Here's how the part is built. I have some questions about the finished solid (model axes, mm). A direction names the side the tool comes from. Give positions to 0.01 mm unless a question says otherwise; leave off trailing zeros. Loops run counter-clockwise (first coordinate to the right, second up) from the corner with the lowest first, then second, coordinate; pieces in that order, holes last.
Q1. Suppose I cut it at C-C (z = 0.6). List the corners of the cut face in (x, y) for me.
Q2. I'm going to push flat-ended pins straight in: P1, Ø3, axis at x = 0, y = -17.5, coming from the -Z side; P2, Ø1, axis at x = -9.5, z = 1, coming from the -Y side. Where does each tip first touch, or does it pass through?
Q3. Suppose I cut it at A-A (y = 0). List the corners of the cut face in (x, z) for me, and give its area (3 significant figures).
Q4. Thinking about a two-plate mould opening in X: for faces 3 (the face through (-4.336, -19.524, 0.493)), 4 (the face through (0, -3, 2)), 5 (the face through (-0.336, 7.487, 0.986)), 6 (the face through (-0.26, -15.517, 0.493)), which applies, pulls with the +X half, pulls with the -X half, needs draft (parallel to the pull), parting line crosses it, or undercut?
Q5. For faces 1 (the face through (1.478, 0.466, 0.986)), 2 (the face through (3, 15, 1)), which set-ups out of +Z, -Z, +X, -X, +Y, -Y let a thin tool reach every point of the face, with its end or its side?
Q6. I need wall thicknesses on probe 1 along Y at (x, z) = (0, 0.4); probe 2 along Y at (x, z) = (0, 1.4); probe 3 along Y at (x, z) = (-0.5, 0.5). Which ranges of each line are inside material? Lowest first, please.
Q7. Suppose I cut it at D-D (x = -9.5). List the corners of the cut face in (y, z) for me.
Q8. Suppose I cut it at B-B (x = 0). List the corners of the cut face in (y, z) for me, and give its area (3 significant figures).
```python
from build123d import *

# Parameters (mm, degrees)
SKETCH1_R           = 20
SKETCH1_R_2         = 15
SKETCH1_R_3         = 2
BOSS_EXTRUDE1_DEPTH = 1
SKETCH1_4_R         = 15
SKETCH1_4_R_2       = 1.55
BOSS_EXTRUDE2_DEPTH = 2


with BuildPart() as part:
    # Sketch1 → Boss-Extrude1 (new body)
    with BuildSketch(Plane(origin=(0, 0, 0), x_dir=(0, 1, 0), z_dir=(0, 0, 1))):
        with Locations(Location((0, 0, 0), (0, 0, 270))):
            Circle(SKETCH1_R)
        with Locations(Location((0, 0, 0), (0, 0, 270))):
            Circle(SKETCH1_R_2, mode=Mode.SUBTRACT)
        with Locations(Location((-17.5, 0, 0), (0, 0, 270))):
            Circle(SKETCH1_R_3, mode=Mode.SUBTRACT)
    extrude(amount=BOSS_EXTRUDE1_DEPTH)

    # Sketch1_4 → Boss-Extrude2 (add)
    with BuildSketch(Plane(origin=(0, 0, 0), x_dir=(0, 1, 0), z_dir=(0, 0, 1))):
        with Locations(Location((0, 0, 0), (0, 0, 270))):
            Circle(SKETCH1_4_R)
        with Locations(Location((9, 0, 0), (0, 0, 270))):
            Circle(SKETCH1_4_R_2, mode=Mode.SUBTRACT)
        with Locations(Location((0, 0, 0), (0, 0, 270))):
            Circle(SKETCH1_4_R_2, mode=Mode.SUBTRACT)
    extrude(amount=BOSS_EXTRUDE2_DEPTH)


solid = part.part
```
Solutions:
1. outline: circle Ø40 at (0, 0); hole circle Ø4 at (0, -17.5); hole circle Ø3.1 at (0, 0); hole circle Ø3.1 at (0, 9)
2. P1: passes through
2. P2: stops at y = -17.86
3. outline: (-20, 0) - (-1.55, 0) - (-1.55, 2) - (-15, 2) - (-15, 1) - (-20, 1) - close; (1.55, 0) - (20, 0) - (20, 1) - (15, 1) - (15, 2) - (1.55, 2) - close
3. area: 63.8 mm2
4. face 3: parting line crosses it
4. face 4: needs draft
4. face 5: undercut
4. face 6: undercut
5. face 1: +Z, -Z
5. face 2: +Z
6. probe 1: y = -20 to -19.5, -15.5 to -1.55, 1.55 to 7.45, 10.55 to 20
6. probe 2: y = -15 to -1.55, 1.55 to 7.45, 10.55 to 15
6. probe 3: y = -19.99 to -19.44, -15.56 to -1.47, 1.47 to 7.53, 10.47 to 19.99
7. outline: (-17.6, 0) - (17.6, 0) - (17.6, 1) - (11.61, 1) - (11.61, 2) - (-11.61, 2) - (-11.61, 1) - (-17.6, 1) - close
8. outline: (-20, 0) - (-19.5, 0) - (-19.5, 1) - (-20, 1) - close; (-15.5, 0) - (-1.55, 0) - (-1.55, 2) - (-15, 2) - (-15, 1) - (-15.5, 1) - close; (1.55, 0) - (7.45, 0) - (7.45, 2) - (1.55, 2) - close; (10.55, 0) - (20, 0) - (20, 1) - (15, 1) - (15, 2) - (10.55, 2) - close
8. area: 53.6 mm2
